Source: CAD feature listing. Evaluate the final solid. Frame: model axes, mm. A direction names the side the tool comes from. Coordinates: 2 decimals unless noted, no trailing zeros. Order: outer loops, then holes, each group sorted by start corner. A loop starts at its lowest first (then second) coordinate and runs counter-clockwise, first axis right, second up.
```python
from build123d import *

# Parameters (mm, degrees)
SKETCH1_W                = 115
SKETCH1_H                = 64
BOSS_EXTRUDE1_DEPTH      = 3
SKETCH2_W                = 115
SKETCH2_H                = 64
SKETCH2_W_2              = 111
SKETCH2_H_2              = 60
BOSS_EXTRUDE2_DEPTH      = 35
BOSS_EXTRUDE9_DEPTH      = 5
BOSS_EXTRUDE9_DEPTH_BACK = 37
SKETCH12_W               = 5
SKETCH12_H               = 5
CUT_EXTRUDE6_DEPTH       = 78.008116455
BOSS_EXTRUDE11_DEPTH     = 10
SKETCH19_W               = 5.5
SKETCH19_H               = 5.5
CUT_EXTRUDE7_DEPTH       = 7
FILLET2_R                = 10
SKETCH20_R               = 15
CUT_EXTRUDE8_DEPTH       = 127.877894056


with BuildPart() as part:
    # Sketch1 → Boss-Extrude1 (new body)
    with BuildSketch(Plane(origin=(0, 0, 0), x_dir=(1, 0, 0), z_dir=(0, 1, 0))):
        Rectangle(SKETCH1_W, SKETCH1_H)
    extrude(amount=BOSS_EXTRUDE1_DEPTH)

    # Sketch2 → Boss-Extrude2 (add)
    with BuildSketch(Plane(origin=(0, 3, 0), x_dir=(1, 0, 0), z_dir=(0, 1, 0))):
        Rectangle(SKETCH2_W, SKETCH2_H)
        Rectangle(SKETCH2_W_2, SKETCH2_H_2, mode=Mode.SUBTRACT)
    extrude(amount=BOSS_EXTRUDE2_DEPTH)

    # Sketch12 → Boss-Extrude9 (add, two sides: drawn at the far end of the back side and taken through both)
    with BuildSketch(Plane(origin=(0, 38, 0), x_dir=(1, 0, 0), z_dir=(0, 1, 0)).offset(-BOSS_EXTRUDE9_DEPTH_BACK)):
        with Locations((-53, 27.5)):
            Rectangle(SKETCH12_W, SKETCH12_H)
        with Locations((53, 27.5)):
            Rectangle(SKETCH12_W, SKETCH12_H)
        with Locations((53, -27.5)):
            Rectangle(SKETCH12_W, SKETCH12_H)
        with Locations((-53, -27.5)):
            Rectangle(SKETCH12_W, SKETCH12_H)
    extrude(amount=BOSS_EXTRUDE9_DEPTH + BOSS_EXTRUDE9_DEPTH_BACK)

    # Sketch14 → Cut-Extrude6 (cut, through all)
    with BuildSketch(Plane(origin=(0, 3, 0), x_dir=(1, 0, 0), z_dir=(0, 1, 0))):
        with BuildLine():
            Line((-53.5, -10), (-53.5, 10))
            ThreePointArc((-53.5, 10), (-48.5, 15), (-43.5, 10))
            Line((-43.5, 10), (-43.5, -10))
            ThreePointArc((-43.5, -10), (-48.5, -15), (-53.5, -10))
        make_face()
    extrude(amount=-CUT_EXTRUDE6_DEPTH, mode=Mode.SUBTRACT)

    # Sketch17 → Boss-Extrude11 (add)
    with BuildSketch(Plane(origin=(0, 3, 0), x_dir=(1, 0, 0), z_dir=(0, 1, 0))):
        Polygon((-45.5, 30), (-50.5, 30), (-50.5, 25), (-55.5, 25), (-55.5, 20), (-45.5, 20), align=None)
        Polygon((50.5, 30), (45.5, 30), (45.5, 20), (55.5, 20), (55.5, 25), (50.5, 25), align=None)
        Polygon((55.5, -25), (55.5, -20), (45.5, -20), (45.5, -30), (50.5, -30), (50.5, -25), align=None)
        Polygon((-45.5, -20), (-55.5, -20), (-55.5, -25), (-50.5, -25), (-50.5, -30), (-45.5, -30), align=None)
    extrude(amount=BOSS_EXTRUDE11_DEPTH)

    # Sketch19 → Cut-Extrude7 (cut)
    with BuildSketch(Plane.XZ):
        with Locations((-52.75, 27.25)):
            Rectangle(SKETCH19_W, SKETCH19_H)
        with Locations((52.75, 27.25)):
            Rectangle(SKETCH19_W, SKETCH19_H)
        with Locations((52.75, -27.25)):
            Rectangle(SKETCH19_W, SKETCH19_H)
        with Locations((-52.75, -27.25)):
            Rectangle(SKETCH19_W, SKETCH19_H)
    extrude(amount=-CUT_EXTRUDE7_DEPTH, mode=Mode.SUBTRACT)

    # Fillet2
    fillet2_edges = [part.edges().sort_by_distance(p)[0] for p in [
        (-45.5, 8, 20),
        (45.5, 8, -20),
        (45.5, 8, 20),
        (-45.5, 8, -20),
    ]]
    fillet(fillet2_edges, radius=FILLET2_R - 0.0001)  # a hair under: the kernel refuses the full size

    # Sketch20 → Cut-Extrude8 (cut, through all)
    with BuildSketch(Plane.ZY.offset(57.5)):
        with Locations((0, 38)):
            Circle(SKETCH20_R)
    extrude(amount=-CUT_EXTRUDE8_DEPTH, mode=Mode.SUBTRACT)


solid = part.part
```
1. Pin query (flat end, axial travel): P1, Ø2.5, axis at y = 40.5, z = 28.5, coming from the -X side; P2, Ø4, axis at x = 39.5, z = 16, coming from the +Y side; P3, Ø2.5, axis at x = -53.5, y = 40, coming from the +Z side. Return the tip coordinate at first contact, or that it passes through.
Findings:
P1: stops at x = -55.5
P2: stops at y = 3
P3: stops at z = 30
2. Draft query along X for faces 1 (the face through (-55.5, 3, 27)), 2 (the face through (-55.5, 40, -27)), 3 (the face through (-55.5, 20, 0)), 4 (the face through (-1, 19, -32)). Return one class per face: released by +X, released by -X, zero draft, split by the parting line, or undercut.
Findings:
face 1: undercut
face 2: released by -X
face 3: undercut
face 4: zero draft
3. Section query D-D on z = 17. Return loops of the section in (x, y).
Findings:
outline: (-57.5, 0) - (57.5, 0) - (57.5, 38) - (55.5, 38) - (55.5, 3) - (-55.5, 3) - (-55.5, 38) - (-57.5, 38) - close
4. Access query for faces 5 (the face through (50, 3, -27)), 6 (the face through (53, 40, -30)), 7 (the face through (50.5, 28, 28)). Directions: +Z, -Z, +X, -X, +Y, -Y. A direction counts if a zero-diameter tool reaches every point of the face in a straight line with its end or side. Return the directions, or none.
Findings:
face 5: -Y
face 6: -Z, +X, -X, +Y
face 7: +Y
5. Section query B-B on y = 29. Return loops of the section in (x, z).
Findings:
outline: (-57.5, -32) - (57.5, -32) - (57.5, -12) - (55.5, -12) - (55.5, -25) - (50.5, -25) - (50.5, -30) - (-50.5, -30) - (-50.5, -25) - (-55.5, -25) - (-55.5, -12) - (-57.5, -12) - close; (-57.5, 12) - (-55.5, 12) - (-55.5, 25) - (-50.5, 25) - (-50.5, 30) - (50.5, 30) - (50.5, 25) - (55.5, 25) - (55.5, 12) - (57.5, 12) - (57.5, 32) - (-57.5, 32) - close
6. Section query A-A on z = 0. Return loops of the section in (x, y), plus the area to 3 significant figures.
Findings:
outline: (-57.5, 0) - (-53.5, 0) - (-53.5, 3) - (-55.5, 3) - (-55.5, 23) - (-57.5, 23) - close; (-43.5, 0) - (57.5, 0) - (57.5, 23) - (55.5, 23) - (55.5, 3) - (-43.5, 3) - close
area: 395 mm2
7. Ray query, line 1 (X direction, y = 27, z = -20); line 2 (X direction, y = 39, z = 27.5); line 3 (Z direction, x = -39, y = 10.5). Return the intervals inside material, ascending.
Findings:
line 1: x = -57.5 to -55.5, 55.5 to 57.5
line 2: x = -55.5 to -50.5, 50.5 to 55.5
line 3: z = -32 to -30, 30 to 32
8. Section query C-C on x = -3. Return loops of the section in (y, z), plus the area to 3 significant figures.
Findings:
outline: (0, -32) - (38, -32) - (38, -30) - (3, -30) - (3, 30) - (38, 30) - (38, 32) - (0, 32) - close
area: 332 mm2
